For this review, take the finished solid that the model builds, in its own axes (mm). Give positions to 0.01 mm unless a question says otherwise; leave off trailing zeros. Loops run counter-clockwise (first coordinate to the right, second up) from the corner with the lowest first, then second, coordinate; pieces in that order, holes last.
```python
from build123d import *

# Parameters (mm, degrees)
F0_W     = 46
F0_H     = 26
F1_DEPTH = 1200
F3_D     = 8


with BuildPart() as f1:
    # F0 (on Top) → F1 (new body)
    with BuildSketch(Plane.XY):
        with BuildLine():
            ThreePointArc((25, 11.5), (23.974874, 13.974874), (21.5, 15))
            Line((21.5, 15), (-21.5, 15))
            ThreePointArc((-21.5, 15), (-23.974874, 13.974874), (-25, 11.5))
            Line((-25, 11.5), (-25, -11.5))
            ThreePointArc((-25, -11.5), (-23.974874, -13.974874), (-21.5, -15))
            Line((-21.5, -15), (21.5, -15))
            ThreePointArc((21.5, -15), (23.974874, -13.974874), (25, -11.5))
            Line((25, -11.5), (25, 11.5))
        make_face()
        Rectangle(F0_W, F0_H, mode=Mode.SUBTRACT)
    extrude(amount=F1_DEPTH)

    # F3 (through all)
    with Locations(Plane.YZ.offset(25)):
        with Locations((0, 800)):
            Hole(F3_D / 2)


solid = f1.part
```
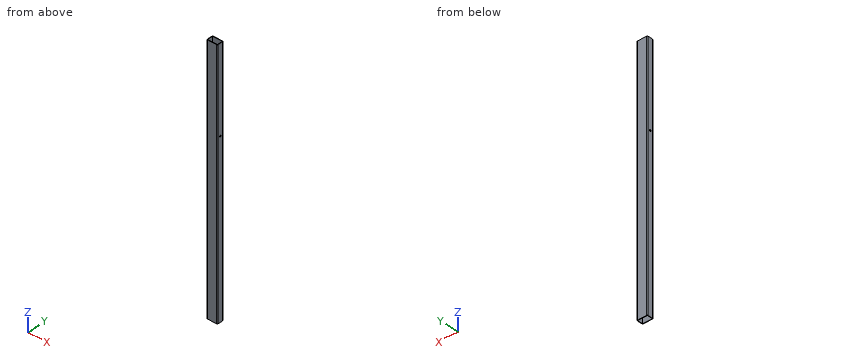
Q1. For pin 1 Ø12 at (x, y) = (-3, -10.5) entering from +Z, flat-tipped, find the tip position at first contact; note if it passes through.
Answers:
pin 1: stops at z = 1200
Q2. Consider section A-A on x = -2.5. Give the boundary of the cut face in (y, z).
Answers:
outline: (-15, 0) - (-13, 0) - (-13, 1200) - (-15, 1200) - close; (13, 0) - (15, 0) - (15, 1200) - (13, 1200) - close
Q3. Consider section B-B on z = 622. Give the boundary of the cut face in (x, y), plus the area to 3 significant figures.
Answers:
outline: (-25, -11.5) arc R3.5 ccw to (-21.5, -15) - (21.5, -15) arc R3.5 ccw to (25, -11.5) - (25, 11.5) arc R3.5 ccw to (21.5, 15) - (-21.5, 15) arc R3.5 ccw to (-25, 11.5) - close; hole (-23, -13) - (23, -13) - (23, 13) - (-23, 13) - close
area: 293 mm2
Q4. For probe 1 along Y at (x, z) = (5, 201); probe 2 along X at (y, z) = (6.5, 50); probe 3 along Z at (x, y) = (-24.6, 0), list the stretches that pass through material, from the lowest coordinate up.
Answers:
probe 1: y = -15 to -13, 13 to 15
probe 2: x = -25 to -23, 23 to 25
probe 3: z = 0 to 796, 804 to 1200
